The listing builds one solid part. Answer for the finished solid, in the listing's coordinates (mm). A direction names the side the tool comes from. Coordinates: 2 decimals unless noted, no trailing zeros. Loops run counter-clockwise (first coordinate to the right, second up) from the corner with the lowest first, then second, coordinate; pieces in that order, holes last. Notation, with made-up numbers: (22.5, -12) - (76.5, -12) arc R16 cw to (76.5, -2) - close; hole circle Ø4 at (14, 37.5). An arc over 180 degrees is marked (long way). One line per question, with ' | ' between items.
from build123d import *

# Parameters (mm, degrees)
ESQUISSE1_W                  = 15.8
ESQUISSE1_H                  = 8
BOSS_EXTRU_1_DEPTH           = 25.01
ESQUISSE2_R                  = 2.4
ENL_V_MAT_EXTRU_1_DEPTH      = 1.7
ESQUISSE3_W                  = 1.9
ESQUISSE3_H                  = 8
ENL_V_MAT_EXTRU_2_DEPTH      = 14.68
CONG_1_R                     = 0.2
ENL_V_MAT_EXTRU_4_DEPTH      = 31.645392802
ENL_V_MAT_EXTRU_4_DEPTH_BACK = 31.645392802


with BuildPart() as part:
    # Esquisse1 → Boss.-Extru.1 (new body)
    with BuildSketch(Plane(origin=(0, 0, 0), x_dir=(1, 0, 0), z_dir=(0, 1, 0))):
        with Locations((7.9, 4)):
            Rectangle(ESQUISSE1_W, ESQUISSE1_H)
    extrude(amount=BOSS_EXTRU_1_DEPTH)

    # Esquisse2 → Enlèv. mat.-Extru.1 (cut)
    with BuildSketch(Plane.XZ):
        with Locations(Location((3.95, -4, 0), (0, 0, 270))):
            Circle(ESQUISSE2_R)
        with Locations(Location((11.85, -4, 0), (0, 0, 270))):
            Circle(ESQUISSE2_R)
    extrude(amount=-ENL_V_MAT_EXTRU_1_DEPTH, mode=Mode.SUBTRACT)

    # Esquisse3 → Enlèv. mat.-Extru.2 (cut)
    with BuildSketch(Plane(origin=(0, 25.01, 0), x_dir=(1, 0, 0), z_dir=(0, 1, 0))):
        with Locations((0.95, 4)):
            Rectangle(ESQUISSE3_W, ESQUISSE3_H)
        with Locations((14.85, 4)):
            Rectangle(ESQUISSE3_W, ESQUISSE3_H)
    extrude(amount=-ENL_V_MAT_EXTRU_2_DEPTH, mode=Mode.SUBTRACT)

    # Congé1
    cong_1_edges = [part.edges().sort_by_distance(p)[0] for p in [
        (3.95, 1.7, -1.6),
        (11.85, 1.7, -1.6),
    ]]
    fillet(cong_1_edges, radius=CONG_1_R)

    # Esquisse5 → Enlèv. mat.-Extru.4 (cut, two sides: drawn at the far end of the back side and taken through both)
    with BuildSketch(Plane.XY.offset(-ENL_V_MAT_EXTRU_4_DEPTH_BACK)):
        with BuildLine():
            Line((2.9, 91.29179457), (2.9, 25.01))
            ThreePointArc((2.9, 25.01), (7.9, 20.01), (12.9, 25.01))
            Line((12.9, 25.01), (12.9, 91.29179457))
            Line((12.9, 91.29179457), (12.9, 223.855383709))
            Line((12.9, 223.855383709), (2.9, 223.855383709))
            Line((2.9, 223.855383709), (2.9, 91.29179457))
        make_face()
    extrude(amount=ENL_V_MAT_EXTRU_4_DEPTH + ENL_V_MAT_EXTRU_4_DEPTH_BACK, mode=Mode.SUBTRACT)


solid = part.part
Item 1: Find section A-A, the plane z = -4. Write down the section's boundary in (x, y), plus the area to 3 significant figures.
Taken from the geometry:
outline: (0, 0) - (1.55, 0) - (1.55, 1.5) arc R0.2 cw to (1.75, 1.7) - (6.15, 1.7) arc R0.2 cw to (6.35, 1.5) - (6.35, 0) - (9.45, 0) - (9.45, 1.5) arc R0.2 cw to (9.65, 1.7) - (14.05, 1.7) arc R0.2 cw to (14.25, 1.5) - (14.25, 0) - (15.8, 0) - (15.8, 10.33) - (13.9, 10.33) - (13.9, 25.01) - (12.9, 25.01) arc R5 cw to (2.9, 25.01) - (1.9, 25.01) - (1.9, 10.33) - (0, 10.33) - close | area: 284 mm2
Item 2: Which of the six approach directions +Z, -Z, +X, -X, +Y, -Y give full straight-line access (tool end or side, diameter ignored) to faces 5 (the face through (8, 0, -4)), 6 (the face through (15, 10.33, -4)), 7 (the face through (15.8, 5, -4)), 8 (the face through (12, 1.7, -4)), 9 (the face through (1, 10.33, -4))?
Taken from the geometry:
face 5: +Z, -Z, +X, -X, -Y | face 6: +Z, -Z, +X, +Y | face 7: +Z, -Z, +X, +Y, -Y | face 8: -Y | face 9: +Z, -Z, -X, +Y
Item 3: The mould has two halves that part along X. Classify faces 1 (the face through (1.9, 18, -4)), 2 (the face through (13.9, 18, -4)), 3 (the face through (8, 10, 0)), 4 (the face through (7.79, 20.01, -4.06)): pulls with the +X half, pulls with the -X half, needs draft (parallel to the pull), parting line crosses it, or undercut.
Taken from the geometry:
face 1: pulls with the -X half | face 2: pulls with the +X half | face 3: needs draft | face 4: undercut
Item 4: Find section C-C, the plane y = 19. Write down the section's boundary in (x, z), plus the area to 3 significant figures.
Taken from the geometry:
outline: (1.9, -8) - (13.9, -8) - (13.9, 0) - (1.9, 0) - close | area: 96.0 mm2
Item 5: Each of these flat-tipped pins is pushed along its axis until it touches: pin 1 Ø2 at (x, z) = (3.5, -3) entering from -Y; pin 2 Ø0.9 at (x, z) = (15, -3.5) entering from +Y; pin 3 Ø1 at (y, z) = (11, -1) entering from +X. Where does it stop, or does it pass through?
Taken from the geometry:
pin 1: stops at y = 1.7 | pin 2: stops at y = 10.33 | pin 3: stops at x = 13.9
Item 6: Find section B-B, the plane x = 11.85. Write down the section's boundary in (y, z), plus the area to 3 significant figures.
Taken from the geometry:
outline: (0, -8) - (21.94, -8) - (21.94, 0) - (0, 0) - (0, -1.6) - (1.5, -1.6) arc R0.2 cw to (1.7, -1.8) - (1.7, -6.2) arc R0.2 cw to (1.5, -6.4) - (0, -6.4) - close | area: 167 mm2
Item 7: Find the intervals of material crossed by line 1 (X direction, y = 1.15, z = -4); line 2 (X direction, y = 13.25, z = -6.75); line 3 (Y direction, x = 1.5, z = -1.5), in increasing order. Write a range as [from, to].
Taken from the geometry:
line 1: x = [0, 1.55], [6.35, 9.45], [14.25, 15.8] | line 2: x = [1.9, 13.9] | line 3: y = [0, 10.33]
Item 8: Find section D-D, the plane z = -1. Write down the section's boundary in (x, y), plus the area to 3 significant figures.
Taken from the geometry:
outline: (0, 0) - (15.8, 0) - (15.8, 10.33) - (13.9, 10.33) - (13.9, 25.01) - (12.9, 25.01) arc R5 cw to (2.9, 25.01) - (1.9, 25.01) - (1.9, 10.33) - (0, 10.33) - close | area: 300 mm2
